```python
from build123d import *

# Parameters (mm, degrees)
F1_DEPTH = 14
F2_R     = 13.3833019173
F3_DEPTH = 2.3


with BuildPart() as f1:
    # F0 (on Top) → F1 (new body)
    with BuildSketch(Plane.XY):
        with BuildLine():
            Line((1.5, 1.5), (9.8868599666, 1.5))
            ThreePointArc((9.8868599666, 1.5), (7.0710678119, 7.0710678119), (1.5, 9.8868599666))
            Line((1.5, 9.8868599666), (1.5, 1.5))
        make_face()
    extrude(amount=F1_DEPTH)



with BuildPart() as f1b:
    # F0 (on Top) → F1, piece 2 (new body)
    with BuildSketch(Plane.XY):
        with BuildLine():
            ThreePointArc((1.5, -9.8868599666), (7.0710678119, -7.0710678119), (9.8868599666, -1.5))
            Line((9.8868599666, -1.5), (1.5, -1.5))
            Line((1.5, -1.5), (1.5, -9.8868599666))
        make_face()
    extrude(amount=F1_DEPTH)


with BuildPart() as f1c:
    # F0 (on Top) → F1, piece 3 (new body)
    with BuildSketch(Plane.XY):
        with BuildLine():
            Line((-1.5, 1.5), (-1.5, 9.8868599666))
            ThreePointArc((-1.5, 9.8868599666), (-7.0710678119, 7.0710678119), (-9.8868599666, 1.5))
            Line((-9.8868599666, 1.5), (-1.5, 1.5))
        make_face()
    extrude(amount=F1_DEPTH)


with BuildPart() as f1d:
    # F0 (on Top) → F1, piece 4 (new body)
    with BuildSketch(Plane.XY):
        with BuildLine():
            ThreePointArc((-9.8868599666, -1.5), (-7.0710678119, -7.0710678119), (-1.5, -9.8868599666))
            Line((-1.5, -9.8868599666), (-1.5, -1.5))
            Line((-1.5, -1.5), (-9.8868599666, -1.5))
        make_face()
    extrude(amount=F1_DEPTH)


with BuildPart() as f1_1:
    add(f1.part)

    add(f1b.part)  # F3 merges F1b

    add(f1c.part)  # F3 merges F1c

    add(f1d.part)  # F3 merges F1d
    # F2 (on face) → F3 (join)
    with BuildSketch(Plane.XY.offset(14)):
        Circle(F2_R)
        with BuildLine():
            Line((-1.5, 1.5), (-9.8868599666, 1.5))
            ThreePointArc((-9.8868599666, 1.5), (-7.0710678119, 7.0710678119), (-1.5, 9.8868599666))
            Line((-1.5, 9.8868599666), (-1.5, 1.5))
        make_face(mode=Mode.SUBTRACT)
        with BuildLine():
            ThreePointArc((-1.5, 9.8868599666), (-7.0710678119, 7.0710678119), (-9.8868599666, 1.5))
            Line((-9.8868599666, 1.5), (-1.5, 1.5))
            Line((-1.5, 1.5), (-1.5, 9.8868599666))
        make_face()
    extrude(amount=F3_DEPTH)


solid = f1_1.part
```
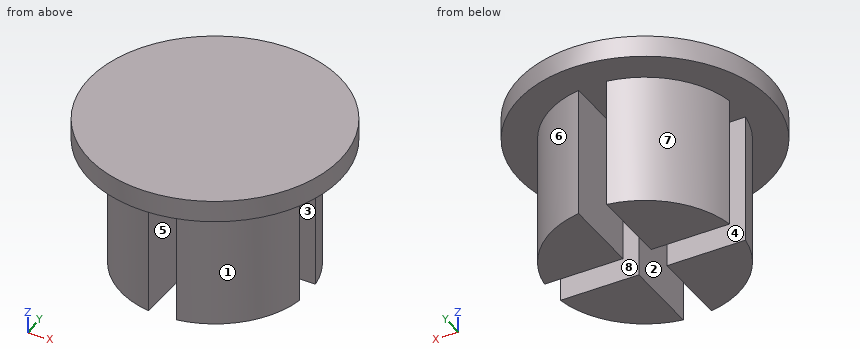
CAD build for the part. Positions are in the model's coordinates, mm. Face numbers are marked on the shaded views. A direction names the side the tool comes from. Coordinates: 2 decimals unless noted, no trailing zeros. Order: outer loops, then holes, each group sorted by start corner. A loop starts at its lowest first (then second) coordinate and runs counter-clockwise, first axis right, second up. Notation, with made-up numbers: M 37,83 L 41,83 A35 ccw 41,122 Z; hole C -21,14.5 d10. An arc over 180 degrees is marked long. Write each question's results on one line, items separated by ' | '. Start each with the question number.
Q1. Flat gauge pins, fed straight in: P1, Ø8, axis at x = -3.5, z = 4.5, coming from the -Y side; P2, Ø2.5, axis at x = 4, z = 10.5, coming from the -Y side; P3, Ø5, axis at x = -6.5, z = 4, coming from the -Y side. Where does each tip first touch, or does it go through?
Q2. Drill centre lines: probe 1 along Z at (x, y) = (-4.5, 0); probe 2 along Y at (x, z) = (5, 1); probe 3 along X at (y, z) = (2.25, 3.5). Where is each one in solid material? Low to high. Write a range as from..to.
Q3. Cut at D-D (x = 0). List the corners of the cut face in (y, z).
Q4. Cut at B-B (x = 4.75). List the corners of the cut face in (y, z), then the cut area to 3 significant figures.
Q5. Which spindle directions (+Z, -Z, +X, -X, +Y, -Y) get a long thin tool onto all of the face, cutting with end or side? Do the marked faces 5, 6, 7 and 8. Say none if no direction does.
Q6. Cut at A-A (z = 8.75). List the corners of the cut face in (x, y).
Q7. Pull direction Y, two halves, no side cores. Call the marked faces 1, 2, 3 and 4: +Y half, -Y half, draft (parallel to the pull), parting line (faces both ways), or undercut.
Q8. Cut at C-C (y = 3.25). List the corners of the cut face in (x, z).
Found:
1) P1: y = -9.89 | P2: y = -9.61 | P3: y = -9.17
2) probe 1: 14..16.3 | probe 2: -8.66..-1.5, 1.5..8.66 | probe 3: -9.74..-1.5, 1.5..9.74
3) outline: M -13.38,14 L 13.38,14 L 13.38,16.3 L -13.38,16.3 Z
4) outline: M -12.51,14 L -8.8,14 L -8.8,0 L -1.5,0 L -1.5,14 L 1.5,14 L 1.5,0 L 8.8,0 L 8.8,14 L 12.51,14 L 12.51,16.3 L -12.51,16.3 Z | area: 262 mm²
5) face 5: -Z, +Y, -Y | face 6: -Z, +X, +Y | face 7: -Z, -X, +Y | face 8: -Z, +X, -X
6) outline: M -9.89,-1.5 A10 ccw -1.5,-9.89 L -1.5,-1.5 Z; M -9.89,1.5 L -1.5,1.5 L -1.5,9.89 A10 ccw Z; M 1.5,-9.89 A10 ccw 9.89,-1.5 L 1.5,-1.5 Z; M 1.5,1.5 L 9.89,1.5 A10 ccw 1.5,9.89 Z
7) face 1: -Y half | face 2: draft | face 3: undercut | face 4: undercut
8) outline: M -12.98,14 L -9.46,14 L -9.46,0 L -1.5,0 L -1.5,14 L 1.5,14 L 1.5,0 L 9.46,0 L 9.46,14 L 12.98,14 L 12.98,16.3 L -12.98,16.3 Z
